from build123d import *

# Parameters (mm, degrees)
SKETCH_1_W      = 12.3
SKETCH_1_H      = 11.3
EXTRUDE_1_DEPTH = 1
SKETCH_2_W      = 1.35
SKETCH_2_H      = 4
SKETCH_2_W_2    = 1.5
EXTRUDE_2_DEPTH = 5.35
SKETCH_3_W      = 1.6
SKETCH_3_H      = 4
EXTRUDE_3_DEPTH = 0.8
SKETCH_4_W      = 1.6
SKETCH_4_H      = 4
EXTRUDE_4_DEPTH = 0.8
FILLET_1_R      = 0.8
FILLET_2_R      = 0.3
SKETCH_5_W      = 1
SKETCH_5_H      = 11.3
EXTRUDE_5_DEPTH = 0.8
SKETCH_6_W      = 1
SKETCH_6_H      = 11.3
EXTRUDE_6_DEPTH = 0.8
FILLET_3_R      = 0.8


with BuildPart() as part:
    # 스케치1 → 보스-돌출1 (new body)
    with BuildSketch(Plane.XY):
        Rectangle(SKETCH_1_W, SKETCH_1_H)
    extrude(amount=EXTRUDE_1_DEPTH)

    # 스케치2 → 보스-돌출2 (add)
    with BuildSketch(Plane.XY.offset(1)):
        with Locations((-5.475, 0)):
            Rectangle(SKETCH_2_W, SKETCH_2_H)
        with Locations((5.4, 0)):
            Rectangle(SKETCH_2_W_2, SKETCH_2_H)
    extrude(amount=EXTRUDE_2_DEPTH)

    # 스케치3 → 보스-돌출3 (add)
    with BuildSketch(Plane(origin=(-4.8, 0, 0), x_dir=(0, 0, -1), z_dir=(1, 0, 0))):
        with Locations((-5.55, 0)):
            Rectangle(SKETCH_3_W, SKETCH_3_H)
    extrude(amount=EXTRUDE_3_DEPTH)

    # 스케치4 → 보스-돌출4 (add)
    with BuildSketch(Plane.ZY.offset(-4.65)):
        with Locations((5.55, 0)):
            Rectangle(SKETCH_4_W, SKETCH_4_H)
    extrude(amount=EXTRUDE_4_DEPTH)

    # 필렛1
    fillet_1_edges = [part.edges().sort_by_distance(p)[0] for p in [
        (3.85, 0, 6.35),
        (3.85, 0, 4.75),
        (-4, 0, 6.35),
        (-4, 0, 4.75),
    ]]
    fillet(fillet_1_edges, radius=FILLET_1_R - 0.0001)  # a hair under: the kernel refuses the full size

    # 필렛2
    fillet_2_edges = [part.edges().sort_by_distance(p)[0] for p in [
        (-4.8, 0, 1),
        (4.65, 0, 1),
    ]]
    fillet(fillet_2_edges, radius=FILLET_2_R)

    # 스케치5 → 보스-돌출5 (add)
    with BuildSketch(Plane.ZY.offset(6.15)):
        with Locations((0.5, 0)):
            Rectangle(SKETCH_5_W, SKETCH_5_H)
    extrude(amount=EXTRUDE_5_DEPTH)

    # 스케치6 → 보스-돌출6 (add)
    with BuildSketch(Plane(origin=(6.15, 0, 0), x_dir=(0, 0, -1), z_dir=(1, 0, 0))):
        with Locations((-0.5, 0)):
            Rectangle(SKETCH_6_W, SKETCH_6_H)
    extrude(amount=EXTRUDE_6_DEPTH)

    # 필렛3
    fillet_3_edges = [part.edges().sort_by_distance(p)[0] for p in [
        (-6.15, 0, 1),
        (6.15, 0, 1),
    ]]
    fillet(fillet_3_edges, radius=FILLET_3_R - 0.0001)  # a hair under: the kernel refuses the full size


solid = part.part
The listing builds one solid part. Answer for the finished solid, in the listing's coordinates (mm). A direction names the side the tool comes from. Coordinates: 2 decimals unless noted, no trailing zeros. Write each loop counter-clockwise with the first axis right and the second up, starting at its lowest first coordinate (ties: lowest second). Pieces come first, ordered by that corner, then holes. Notation, with made-up numbers: M -39,71 L 14,71 A16 ccw 14,91 Z; hole C -12,-25 d11. An arc over 180 degrees is marked long. Use one line per item in the form item = value.
Item 1: Given P1, Ø3, axis at x = -5.5, z = 4.5, coming from the +Y side; P2, Ø2, axis at y = -1, z = 4, coming from the -X side; P3, Ø3, axis at y = -1, z = 4, coming from the +X side; P4, Ø3, axis at x = 0.5, z = 5.5, coming from the +Y side, each flat-ended and moving along its own axis, determine where each tip first touches the part or whether it passes through.
Model answer:
P1 = 2
P2 = -6.15
P3 = 6.15
P4 = through
Item 2: Find section A-A, the plane z = 2.5. Give the vertices of the cut face in (x, y).
Model answer:
outline = M -6.15,-2 L -4.8,-2 L -4.8,2 L -6.15,2 Z; M 4.65,-2 L 6.15,-2 L 6.15,2 L 4.65,2 Z
Item 3: Find section C-C, the plane x = 5. Give the vertices of the cut face in (y, z).
Model answer:
outline = M -5.65,0 L 5.65,0 L 5.65,1 L 2,1 L 2,6.35 L -2,6.35 L -2,1 L -5.65,1 Z
Item 4: The mould has two halves that part along Z. Classify faces 1 (the face through (4.65, 0, 3)), 2 (the face through (5, -2, 4)), 3 (the face through (0, 0, 0)): released by +Z, released by -Z, zero draft, split by the parting line, or undercut.
Model answer:
face_1 = undercut
face_2 = zero draft
face_3 = released by -Z
Item 5: Find section D-D, the plane z = 5.75. Give the vertices of the cut face in (x, y).
Model answer:
outline = M -6.15,-2 L -4.03,-2 L -4.03,2 L -6.15,2 Z; M 3.88,-2 L 6.15,-2 L 6.15,2 L 3.88,2 Z
Item 6: Find the intervals of material crossed by probe 1 along X at (y, z) = (0, 4); probe 2 along X at (y, z) = (-1, 5.5); probe 3 along Z at (x, y) = (6.25, 2.25), in increasing order.
Model answer:
probe_1 = -6.15 to -4.8, 4.65 to 6.15
probe_2 = -6.15 to -4, 3.85 to 6.15
probe_3 = 0 to 1
Item 7: For faces 4 (the face through (-5, -2, 4)), 5 (the face through (-6.15, 0, 4)), 6 (the face through (5, 2, 4)), determine the directions among +Z, -Z, +X, -X, +Y, -Y from which every point of the face is accessible in a straight line to the end or side of a thin tool.
Model answer:
face_4 = +Z, +X, -X, -Y
face_5 = +Z, -X, +Y, -Y
face_6 = +Z, +X, -X, +Y
